```python
from build123d import *

# Parameters (mm, degrees)
SKETCH2_W           = 460
SKETCH2_H           = 700
SKETCH2_W_2         = 305
SKETCH2_H_2         = 600
BOSS_EXTRUDE1_DEPTH = 20
SKETCH10_W          = 460
SKETCH10_H          = 700
BOSS_EXTRUDE6_DEPTH = 20
SKETCH11_W          = 30
SKETCH11_H          = 30
BOSS_EXTRUDE7_DEPTH = 180
SKETCH14_W          = 40
SKETCH14_H          = 352
BOSS_EXTRUDE8_DEPTH = 40
SKETCH15_W          = 30
SKETCH15_H          = 30
BOSS_EXTRUDE9_DEPTH = 180
SKETCH17_R          = 26
CUT_EXTRUDE1_DEPTH  = 60
CUT_EXTRUDE2_DEPTH  = 20


with BuildPart() as part:
    # Sketch2 → Boss-Extrude1 (new body)
    with BuildSketch(Plane(origin=(0, 0, 0), x_dir=(1, 0, 0), z_dir=(0, 1, 0))):
        with Locations((230, 350)):
            Rectangle(SKETCH2_W, SKETCH2_H)
        with Locations((212.5, 350)):
            Rectangle(SKETCH2_W_2, SKETCH2_H_2, mode=Mode.SUBTRACT)
    extrude(amount=BOSS_EXTRUDE1_DEPTH)

    # Sketch10 → Boss-Extrude6 (add)
    with BuildSketch(Plane.XZ):
        with Locations((230, -350)):
            Rectangle(SKETCH10_W, SKETCH10_H)
    extrude(amount=BOSS_EXTRUDE6_DEPTH)

    # Sketch11 → Boss-Extrude7 (add)
    with BuildSketch(Plane.XZ.offset(20)):
        with Locations((15, -15)):
            Rectangle(SKETCH11_W, SKETCH11_H)
        with Locations((445, -15)):
            Rectangle(SKETCH11_W, SKETCH11_H)
        with Locations((15, -685)):
            Rectangle(SKETCH11_W, SKETCH11_H)
        with Locations((445, -685)):
            Rectangle(SKETCH11_W, SKETCH11_H)
    extrude(amount=BOSS_EXTRUDE7_DEPTH)

    # Sketch14 → Boss-Extrude8 (add)
    with BuildSketch(Plane(origin=(0, 20, 0), x_dir=(1, 0, 0), z_dir=(0, 1, 0))):
        with Locations((20, 876)):
            Rectangle(SKETCH14_W, SKETCH14_H)
        with Locations((440, 876)):
            Rectangle(SKETCH14_W, SKETCH14_H)
    extrude(amount=-BOSS_EXTRUDE8_DEPTH)

    # Sketch15 → Boss-Extrude9 (add)
    with BuildSketch(Plane.XZ.offset(20)):
        with Locations((445, -1037)):
            Rectangle(SKETCH15_W, SKETCH15_H)
        with Locations((15, -1037)):
            Rectangle(SKETCH15_W, SKETCH15_H)
    extrude(amount=BOSS_EXTRUDE9_DEPTH)

    # Sketch17 → Cut-Extrude1 (cut)
    with BuildSketch(Plane(origin=(0, 20, 0), x_dir=(1, 0, 0), z_dir=(0, 1, 0))):
        with BuildLine():
            Line((365, 650), (339, 650))
            ThreePointArc((339, 650), (346.615223689, 631.615223689), (365, 624))
            Line((365, 624), (365, 650))
        make_face()
        with BuildLine():
            ThreePointArc((391, 650), (365, 676), (339, 650))
            Line((339, 650), (365, 650))
            Line((365, 650), (365, 624))
            ThreePointArc((365, 624), (383.384776311, 631.615223689), (391, 650))
        make_face()
        with BuildLine():
            Line((365, 324), (365, 376))
            ThreePointArc((365, 376), (339, 350), (365, 324))
        make_face()
        with BuildLine():
            ThreePointArc((391, 350), (383.384776311, 368.384776311), (365, 376))
            Line((365, 376), (365, 324))
            ThreePointArc((365, 324), (383.384776311, 331.615223689), (391, 350))
        make_face()
        with BuildLine():
            Line((365, 50), (365, 76))
            ThreePointArc((365, 76), (346.615223689, 68.384776311), (339, 50))
            Line((339, 50), (365, 50))
        make_face()
        with BuildLine():
            ThreePointArc((391, 50), (383.384776311, 68.384776311), (365, 76))
            Line((365, 76), (365, 50))
            Line((365, 50), (339, 50))
            ThreePointArc((339, 50), (365, 24), (391, 50))
        make_face()
        with BuildLine():
            Line((60, 324), (60, 376))
            ThreePointArc((60, 376), (34, 350), (60, 324))
        make_face()
        with BuildLine():
            ThreePointArc((86, 350), (78.384776311, 368.384776311), (60, 376))
            Line((60, 376), (60, 324))
            ThreePointArc((60, 324), (78.384776311, 331.615223689), (86, 350))
        make_face()
        with BuildLine():
            Line((60, 50), (60, 76))
            ThreePointArc((60, 76), (41.615223689, 31.615223689), (86, 50))
            Line((86, 50), (60, 50))
        make_face()
        with BuildLine():
            ThreePointArc((86, 50), (78.384776311, 68.384776311), (60, 76))
            Line((60, 76), (60, 50))
            Line((60, 50), (86, 50))
        make_face()
        with Locations((60, 650)):
            Circle(SKETCH17_R)
    extrude(amount=-CUT_EXTRUDE1_DEPTH, mode=Mode.SUBTRACT)

    # Sketch18 → Cut-Extrude2 (cut)
    with BuildSketch(Plane(origin=(0, 20, 0), x_dir=(1, 0, 0), z_dir=(0, 1, 0))):
        Polygon((60, 700), (365, 700), (365, 650), (212.5, 650), (60, 650), align=None)
    extrude(amount=-CUT_EXTRUDE2_DEPTH, mode=Mode.SUBTRACT)


solid = part.part
```
Check sheet for the modelled part. Datum: model origin and axes. Units: mm. A direction names the side the tool comes from. Round coordinates to 2 decimals unless told otherwise and drop trailing zeros. Order: outer loops, then holes, each group sorted by start corner. A loop starts at its lowest first (then second) coordinate and runs counter-clockwise, first axis right, second up. Notation, with made-up numbers: (-27.75, 74) - (-19.75, 74) arc R17 cw to (-19.75, 97) - close; hole circle Ø5 at (5, 88.5). An arc over 180 degrees is marked (long way). Answer as CSV lines item,"result". Start each with the question number.
1) Draft check along Z on faces 5 (the face through (15, -109, -670)), 6 (the face through (444, -88, -1052)), 7 (the face through (15, -200, -685)), 8 (the face through (34.025, -4.164, -651.143)). Enter one of: +Z half, -Z half, draft (parallel to the pull), parting line (faces both ways), or undercut.
2) Section check D-D (z = -506). Record the cut outline in (x, y), then the cut area to 3 significant figures.
3) Section check B-B (z = -792.5). Record the cut outline in (x, y).
4) Depth check by flat-ended pin: pin 1 (6 mm diameter, centred on x = 318, z = -128, fed in from -Y); pin 2 (24 mm diameter, centred on y = -143, z = -679.5, fed in from -X). Enter the tip coordinate at first touch or a pass-through.
5) Section check A-A (y = -155.5). Record the cut outline in (x, z).
6) Section check C-C (x = 381.5). Record the cut outline in (y, z).
7) Scan lines: probe 1 along Z at (x, y) = (60, -4); probe 2 along X at (y, z) = (5.5, -650); probe 3 along X at (y, z) = (-1, -50). Record each from-to range of solid material in increasing order.
8) Tool access check on faces 1 (the face through (211, 10, -50)), 2 (the face through (445, -109, -1022)), 3 (the face through (30, -109, -685)), 4 (the face through (365.2, 20, -411.6)). Record the directions out of +Z, -Z, +X, -X, +Y, -Y that give a thin tool (end or side, any length) a straight path to the whole face; none if there is none.
Determined:
1,face 5,"undercut"
1,face 6,"-Z half"
1,face 7,"draft"
1,face 8,"undercut"
2,outline,"(0, -20) - (460, -20) - (460, 20) - (365, 20) - (365, 0) - (60, 0) - (60, 20) - (0, 20) - close"
2,area,"12,300 mm^2"
3,outline,"(0, -20) - (40, -20) - (40, 20) - (0, 20) - close; (420, -20) - (460, -20) - (460, 20) - (420, 20) - close"
4,pin 1,"y = -20"
4,pin 2,"x = 0"
5,outline,"(0, -1052) - (30, -1052) - (30, -1022) - (0, -1022) - close; (0, -700) - (30, -700) - (30, -670) - (0, -670) - close; (0, -30) - (30, -30) - (30, 0) - (0, 0) - close; (430, -1052) - (460, -1052) - (460, -1022) - (430, -1022) - close; (430, -700) - (460, -700) - (460, -670) - (430, -670) - close; (430, -30) - (460, -30) - (460, 0) - (430, 0) - close"
6,outline,"(-20, -700) - (20, -700) - (20, -670.09) - (-20, -670.09) - close; (-20, -629.91) - (20, -629.91) - (20, -370.09) - (-20, -370.09) - close; (-20, -329.91) - (20, -329.91) - (20, -70.09) - (-20, -70.09) - close; (-20, -29.91) - (20, -29.91) - (20, 0) - (-20, 0) - close"
7,probe 1,"-700 to -676, -624 to -376, -324 to -76, -24 to 0"
7,probe 2,"0 to 34, 391 to 460"
7,probe 3,"0 to 34, 86 to 339, 391 to 460"
8,face 1,"-Z, +Y"
8,face 2,"+X, -X, -Y"
8,face 3,"+Z, -Z, -Y"
8,face 4,"+Z, -Z, +X, -X, +Y"
